The listing builds one solid part. Answer for the finished solid, in the listing's coordinates (mm). Round coordinates to 2 decimals unless told otherwise and drop trailing zeros. Write each loop counter-clockwise with the first axis right and the second up, starting at its lowest first coordinate (ties: lowest second). Pieces come first, ordered by that corner, then holes. Notation, with made-up numbers: (-10.5, -11.75) - (45.5, -11.75) arc R25 ccw to (45.5, 16.25) - close; hole circle Ø1 at (-23.75, 15.25). An arc over 180 degrees is marked (long way). Return JSON: item names as keys, results as strings. Group by question number.
(1) Section B-B, the plane z = 2 is taken. Write down the section's boundary in (x, y), then the cut area to 3 significant figures.
(2) Find the intervals of material crossed by line 1 along X through (y, z) = (-0.5, 26); line 2 along Z through (x, y) = (-1.25, 4); line 3 along Y through (x, z) = (0.75, -105), in increasing order. Write a range as [from, to].
(3) Section A-A, the plane y = 1.5 is taken. Write down the section's boundary in (x, z), then the cut area to 3 significant figures.
(4) Each of these flat-tipped pins is pushed along its axis until it touches: pin 1 (1.5 mm diameter, centred on y = -2, z = -73, fed in from -X); pin 2 (2.5 mm diameter, centred on y = 1, z = 176, fed in from +X); pin 3 (2.5 mm diameter, centred on x = 1.5, z = -176.5, fed in from -Y). Where does it stop, or does it pass through?
(5) Section C-C, the plane x = 0.75 is taken. Write down the section's boundary in (y, z), then the cut area to 3 significant figures.
```python
from build123d import *

# Parameters (mm, degrees)
SKETCH1_R           = 5
BOSS_EXTRUDE1_DEPTH = 175
SKETCH2_W           = 6
SKETCH2_H           = 6
BOSS_EXTRUDE2_DEPTH = 3


with BuildPart() as part:
    # Sketch1 → Boss-Extrude1 (new, symmetric)
    with BuildSketch(Plane.XY):
        Circle(SKETCH1_R)
    extrude(amount=BOSS_EXTRUDE1_DEPTH, both=True)

    # Sketch2 → Boss-Extrude2 (add)
    with BuildSketch(Plane.XY.offset(175)):
        Rectangle(SKETCH2_W, SKETCH2_H)
    boss_extrude2 = extrude(amount=BOSS_EXTRUDE2_DEPTH)

    # Mirror1: Boss-Extrude2 across plane
    add(boss_extrude2.mirror(Plane.XY))


solid = part.part
```
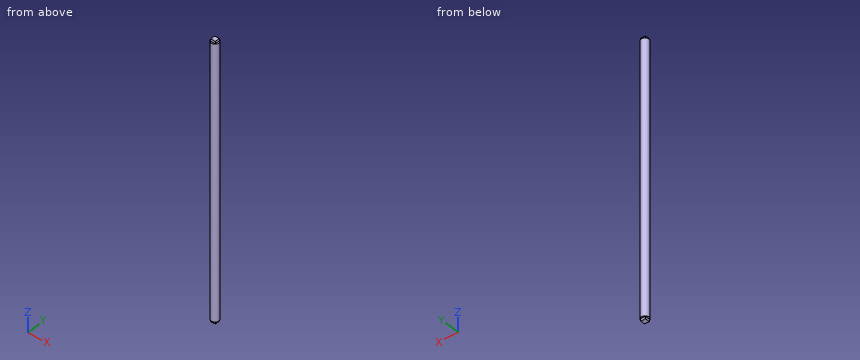
Working result:
{
 "1": {"outline": "circle Ø10 at (0, 0)", "area": "78.5 mm^2"},
 "2": {"line 1": "x = [-4.97, 4.97]", "line 2": "z = [-175, 175]", "line 3": "y = [-4.94, 4.94]"},
 "3": {"outline": "(-4.77, -175) - (-3, -175) - (-3, -178) - (3, -178) - (3, -175) - (4.77, -175) - (4.77, 175) - (3, 175) - (3, 178) - (-3, 178) - (-3, 175) - (-4.77, 175) - close", "area": "3,370 mm^2"},
 "4": {"pin 1": "stops at x = -4.84", "pin 2": "stops at x = 4.99", "pin 3": "stops at y = -3"},
 "5": {"outline": "(-4.94, -175) - (-3, -175) - (-3, -178) - (3, -178) - (3, -175) - (4.94, -175) - (4.94, 175) - (3, 175) - (3, 178) - (-3, 178) - (-3, 175) - (-4.94, 175) - close", "area": "3,500 mm^2"}
}
